Here's how the part is built. I have some questions about the finished solid (model axes, mm). A direction names the side the tool comes from. Coordinates: 2 decimals unless noted, no trailing zeros. Write each loop counter-clockwise with the first axis right and the second up, starting at its lowest first coordinate (ties: lowest second). Pieces come first, ordered by that corner, then holes.
(1) Which directions (+Z, -Z, +X, -X, +Y, -Y) give clear straight access to the entire face, cutting with the end or side of a thin tool? Please do faces 5 (the flat face through (-1, 5, -22.5)), 6 (the flat face through (0.953, -4, -1)), 7 (the flat face through (-2.047, -5, -1)).
(2) Imagine slicing it at B-B, the plane x = -4.35. List the corners of the cut face in (y, z) for me, plus the area to 3 significant figures.
(3) Imagine slicing it at D-D, the plane z = -8.5. List the corners of the cut face in (x, y) for me.
(4) Thinking about a two-plate mould opening in Y: for faces 1 (the cylindrical face through (-0.5, -7.7, -21)), 2 (the flat face through (-1, -2, -37.5)), 3 (the flat face through (-1, 3.277, -15)), 4 (the cylindrical face through (-4.237, 8.407, -30.105)), which applies, released by +Y, released by -Y, zero draft, split by the parting line, or undercut?
(5) Imagine slicing it at A-A, the plane z = 0. List the corners of the cut face in (x, y) for me, plus the area to 3 significant figures.
(6) Imagine slicing it at C-C, the plane y = -2.75. List the corners of the cut face in (x, z) for me.
(7) Please list where these lines run through material, in increasing order: probe 1 along Z at (x, y) = (-2.35, 8); probe 2 along X at (y, z) = (-5.25, -24); probe 3 along Y at (x, z) = (0.35, 0).
(8) For pin 1 Ø3.5 at (y, z) = (-7.64, 22.5) entering from -X; pin 2 Ø2.5 at (x, z) = (-0.5, -17) entering from +Y; pin 3 Ø10 at (y, z) = (-1, -3.5) entering from -X, each with a flat end and sliding along its axis, tell me the tip position at first contact or that it passes through.
```python
from build123d import *

# Parameters (mm, degrees)
BOSS_EXTRUDE1_DEPTH      = 37.5
BOSS_EXTRUDE1_DEPTH_BACK = 37.5
SKETCH2_R                = 1.5
CUT_EXTRUDE3_DEPTH       = 10
CUT_EXTRUDE3_DEPTH_BACK  = 10
SKETCH4_R                = 1.5
SKETCH4_W                = 15
SKETCH4_H                = 10


with BuildPart() as part:
    # Sketch2 → Boss-Extrude1 (new, two sides: drawn at the far end of the back side and taken through both)
    with BuildSketch(Plane.XY.offset(-BOSS_EXTRUDE1_DEPTH_BACK)):
        with BuildLine():
            Line((-2.046544696, -13.643631305), (-2.046544696, 3.356368695))
            ThreePointArc((-2.046544696, 3.356368695), (-4.167865039, 8.477689038), (0.953455304, 6.356368695))
            Line((0.953455304, 6.356368695), (0.953455304, -13.643631305))
            Line((0.953455304, -13.643631305), (-2.046544696, -13.643631305))
        make_face()
        with Locations((-2.046544696, 6.356368695)):
            Circle(SKETCH2_R, mode=Mode.SUBTRACT)
    extrude(amount=BOSS_EXTRUDE1_DEPTH + BOSS_EXTRUDE1_DEPTH_BACK)

    # Sketch4 → Cut-Extrude3 (cut, two sides: drawn at the far end of the back side and taken through both)
    with BuildSketch(Plane.ZY.offset(2.046544696).offset(-CUT_EXTRUDE3_DEPTH_BACK)):
        with Locations(Location((-22.5, -7.643631305, 0), (0, 0, 180))):
            Circle(SKETCH4_R)
        with Locations(Location((0, -7.643631305, 0), (0, 0, 180))):
            Circle(SKETCH4_R)
        with Locations(Location((22.5, -7.643631305, 0), (0, 0, 180))):
            Circle(SKETCH4_R)
        with Locations((-15, 8.277390495)):
            Rectangle(SKETCH4_W, SKETCH4_H)
        with Locations((15, 8.251)):
            Rectangle(SKETCH4_W, SKETCH4_H)
    extrude(amount=CUT_EXTRUDE3_DEPTH + CUT_EXTRUDE3_DEPTH_BACK, mode=Mode.SUBTRACT)


solid = part.part
```
Recorded:
1. face 5: +X, -X, +Y
1. face 6: +Z, -Z, +X, +Y, -Y
1. face 7: +Z, -Z, -X, -Y
2. outline: (4.43, -37.5) - (8.28, -37.5) - (8.28, -22.5) - (4.43, -22.5) - close; (4.43, -7.5) - (8.28, -7.5) - (8.28, 7.5) - (4.43, 7.5) - close; (4.43, 22.5) - (8.28, 22.5) - (8.28, 37.5) - (4.43, 37.5) - close
2. area: 173 mm2
3. outline: (-2.05, -13.64) - (0.95, -13.64) - (0.95, 3.28) - (-2.05, 3.28) - close
4. face 1: undercut
4. face 2: zero draft
4. face 3: released by +Y
4. face 4: split by the parting line
5. outline: (-2.05, -13.64) - (0.95, -13.64) - (0.95, -9.14) - (-2.05, -9.14) - close; (-2.05, -6.14) - (0.95, -6.14) - (0.95, 6.36) arc R3 ccw (long way) to (-2.05, 3.36) - close; hole circle Ø3 at (-2.05, 6.36)
5. area: 65.1 mm2
6. outline: (-2.05, -37.5) - (0.95, -37.5) - (0.95, 37.5) - (-2.05, 37.5) - close
7. probe 1: z = -37.5 to -22.5, -7.5 to 7.5, 22.5 to 37.5
7. probe 2: x = -2.05 to 0.95
7. probe 3: y = -13.64 to -9.14, -6.14 to 8.16
8. pin 1: stops at x = -2.05
8. pin 2: stops at y = 3.28
8. pin 3: stops at x = -3.9
